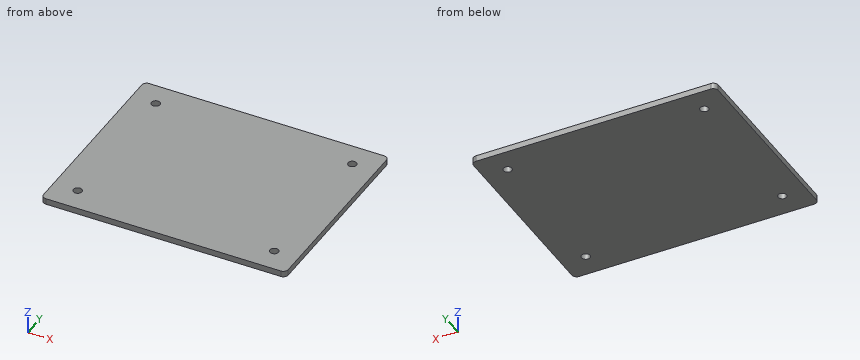
from build123d import *

# Parameters (mm, degrees)
SKETCH_1_W      = 90
SKETCH_1_H      = 70
SKETCH_1_R      = 1.75
EXTRUDE_1_DEPTH = 2.5
SKETCH_2_W      = 102
SKETCH_2_H      = 82
SKETCH_2_W_2    = 90
SKETCH_2_H_2    = 70
EXTRUDE_2_DEPTH = 2.5
FILLET_1_R      = 2


with BuildPart() as part:
    # 草圖1 → 填料-伸長1 (new body)
    with BuildSketch(Plane.XY):
        Rectangle(SKETCH_1_W, SKETCH_1_H)
        with Locations((-41, 31)):
            Circle(SKETCH_1_R, mode=Mode.SUBTRACT)
        with Locations(Location((41, 31, 0), (0, 0, 180))):
            Circle(SKETCH_1_R, mode=Mode.SUBTRACT)
        with Locations((41, -31)):
            Circle(SKETCH_1_R, mode=Mode.SUBTRACT)
        with Locations(Location((-41, -31, 0), (0, 0, 180))):
            Circle(SKETCH_1_R, mode=Mode.SUBTRACT)
    extrude(amount=EXTRUDE_1_DEPTH)

    # 草圖2 → 填料-伸長2 (add)
    with BuildSketch(Plane.XY.offset(2.5)):
        Rectangle(SKETCH_2_W, SKETCH_2_H)
        Rectangle(SKETCH_2_W_2, SKETCH_2_H_2, mode=Mode.SUBTRACT)
    extrude(amount=-EXTRUDE_2_DEPTH)

    # 圓角1
    fillet_1_edges = [part.edges().sort_by_distance(p)[0] for p in [
        (-51, -41, 1.25),
        (-51, 41, 1.25),
        (51, 41, 1.25),
        (51, -41, 1.25),
    ]]
    fillet(fillet_1_edges, radius=FILLET_1_R)


solid = part.part
CAD build for the part. Positions are in the model's coordinates, mm. Coordinates: 2 decimals unless noted, no trailing zeros. Loops run counter-clockwise (first coordinate to the right, second up) from the corner with the lowest first, then second, coordinate; pieces in that order, holes last. Notation, with made-up numbers: (85.5, 85.5) -> (108.5, 85.5) arc R9 ccw to (108.5, 102.5) -> close; hole circle Ø2 at (40, 67). An arc over 180 degrees is marked (long way). One line per item, written item: value.
1. Drill centre lines: line 1 (Y direction, x = -41, z = 1.45); line 2 (X direction, y = 32, z = 0.55). Where is each one in solid material? Low to high. Write a range as [from, to].
Answers:
line 1: y = [-41, -32.75], [-29.25, 29.25], [32.75, 41]
line 2: x = [-51, -42.44], [-39.56, 39.56], [42.44, 51]
2. Flat gauge pins, fed straight in: P1, Ø1, axis at x = 31, y = -22.5, coming from the -Z side; P2, Ø3, axis at x = -41, y = -31, coming from the +Z side. Where does each tip first touch, or does it go through?
Answers:
P1: stops at z = 0
P2: passes through
3. Slice it at A-A on x = -41. Write the cut outline in (y, z), and give its area (4 significant figures).
Answers:
outline: (-41, 0) -> (-32.75, 0) -> (-32.75, 2.5) -> (-41, 2.5) -> close; (-29.25, 0) -> (29.25, 0) -> (29.25, 2.5) -> (-29.25, 2.5) -> close; (32.75, 0) -> (41, 0) -> (41, 2.5) -> (32.75, 2.5) -> close
area: 187.5 mm^2
4. Slice it at B-B on y = -31. Write the cut outline in (x, z), and give its area (4 significant figures).
Answers:
outline: (-51, 0) -> (-42.75, 0) -> (-42.75, 2.5) -> (-51, 2.5) -> close; (-39.25, 0) -> (39.25, 0) -> (39.25, 2.5) -> (-39.25, 2.5) -> close; (42.75, 0) -> (51, 0) -> (51, 2.5) -> (42.75, 2.5) -> close
area: 237.5 mm^2
